Can you work these out from the model? Positions are in its coordinate system, mm. A direction names the side the tool comes from. Give positions to 0.01 mm unless a question says otherwise; leave off trailing zeros. Loops run counter-clockwise (first coordinate to the right, second up) from the corner with the lowest first, then second, coordinate; pieces in that order, holes last. Notation, with made-up numbers: (67.5, -13.5) - (77.5, -13.5) arc R24 ccw to (77.5, 1.5) - close; hole circle Ø5 at (73.25, 72). An arc over 180 degrees is marked (long way). Answer in a Markdown table with one row per item.
Autodesk Inventor part; units mm, degrees
ref_plane "YZ Plane" through (0, 0, 0) normal (1, 0, 0) x (0, 1, 0)
ref_plane "XZ Plane" through (0, 0, 0) normal (0, 1, 0) x (-1, 0, 0)
ref_plane "XY Plane" through (0, 0, 0) normal (0, 0, 1) x (1, 0, 0)
sketch "Sketch1" plane through (0, 0, 0) normal (1, 0, 0) x (0, 1, 0)
  line L0 (0, -278.2902) -> (0, 46.3817) construction
  line L1 (36.388, -206.3665) -> (0, 0) construction
  arc A0 (16.0424, -209.8254) -> (49.6755, -222.1573) centre (36.388, -206.3665) ccw
  line L2 (61.8586, -134.906) -> (45.7568, -169.4363) construction
  arc A1 (66.5803, -134.2844) -> (59.0717, -131.044) centre (61.8586, -134.906) ccw
  arc A2 (73.3134, -202.2667) -> (74.9688, -198.001) centre (70.247, -198.6226) ccw
  arc A3 (11.22, -165.5743) -> (9.3117, -170.2345) centre (14.0068, -169.4363) ccw
  line L3 (66.5803, -134.2844) -> (74.9688, -198.001)
  line L4 (73.3134, -202.2667) -> (49.6755, -222.1573)
  line L5 (16.0424, -209.8254) -> (9.3117, -170.2345)
  line L6 (70.247, -198.6226) -> (45.7568, -169.4363) construction
  line L7 (59.0717, -131.044) -> (11.22, -165.5743)
  line L8 (45.7568, -169.4363) -> (14.0068, -169.4363) construction
  dimension "d8" = 209.55
  dimension "d9" = 175.506
  dimension "d11" = 10
  dimension "d12" = 20.6375
  dimension "d13" = 38.1
  dimension "d14" = 25
  dimension "d19" = 4.7625
  dimension "d37" = 40
  dimension "d39" = 90
  dimension "d40" = 31.75
  dimension "d41" = 38.1
extrude "Plate1" add sketch "Sketch1" along normal blind 3.175
hole "Hole1" at (0, 61.8586, -134.906) at (0, 14.0068, -169.4363) at (0, 70.247, -198.6226) direction (1, 0, 0) diameter 4.9784 end through all
hole "Hole2" at (0, 36.388, -206.3665) at (0, 45.7568, -169.4363) direction (1, 0, 0) diameter 28.575 end through all
sketch "Sketch2" plane through (3.175, 0, 0) normal (1, 0, 0) x (0, 0, -1)
  circle A0 centre (169.4363, 45.7568) radius 14.2875
  circle A1 centre (206.3665, 36.388) radius 14.2875
  circle A2 centre (198.6226, 70.247) radius 2.4892
  circle A3 centre (169.4363, 14.0068) radius 2.4892
  circle A4 centre (134.906, 61.8586) radius 2.4892
  arc A5 (134.2844, 66.5803) -> (131.044, 59.0717) centre (134.906, 61.8586) ccw
  line L0 (165.5743, 11.22) -> (131.044, 59.0717)
  arc A6 (165.5743, 11.22) -> (170.2345, 9.3117) centre (169.4363, 14.0068) ccw
  line L1 (209.8254, 16.0424) -> (170.2345, 9.3117)
  arc A7 (209.8254, 16.0424) -> (222.1573, 49.6755) centre (206.3665, 36.388) ccw
  line L2 (202.2667, 73.3134) -> (222.1573, 49.6755)
  arc A8 (202.2667, 73.3134) -> (198.001, 74.9688) centre (198.6226, 70.247) ccw
  line L3 (134.2844, 66.5803) -> (198.001, 74.9688)
  line L4 (134.906, 61.8586) -> (198.6226, 70.247)
  line L5 (198.6226, 70.247) -> (218.5132, 46.6091)
  arc A9 (209.0271, 20.7375) -> (218.5132, 46.6091) centre (206.3665, 36.388) ccw
  line L6 (209.0271, 20.7375) -> (169.4363, 14.0068)
  line L7 (169.4363, 14.0068) -> (134.906, 61.8586)
  circle A10 centre (134.906, 61.8586) radius 4.7625
  circle A11 centre (198.6226, 70.247) radius 4.7625
  circle A12 centre (169.4363, 14.0068) radius 4.7625
  circle A13 centre (169.4363, 45.7568) radius 22.225
  circle A14 centre (206.3665, 36.388) radius 20.6375
  point P0 (0, 0)
  point P1 (196.0269, 18.5274)
  point P2 (186.3547, 31.3444)
  point P3 (161.5078, 24.9941)
  point P4 (166.6495, 17.8688)
  point P5 (174.1315, 14.805)
  point P6 (191.1791, 50.3612)
  point P7 (210.0229, 56.699)
  point P8 (201.689, 66.603)
  point P9 (193.9009, 69.6254)
  point P10 (175.3438, 67.1823)
  point P11 (147.233, 44.776)
  point P12 (158.1848, 64.9233)
  point P13 (139.6278, 62.4802)
  point P14 (137.6928, 57.9966)
  dimension "d42" = 4.7625
  dimension "d44" = 41.275
  dimension "d45" = 44.45
extrude "Cut1" cut sketch "Sketch2" against normal blind 3.175 contours A11 L5 A14 A13 L4 | A13 L7 A10 L4 | A14 L6 A12 L7 A13
fillet "Corner Round1" radius 1.5875 14 edges at (1.5875, 44.776, -147.233) (1.5875, 64.9233, -158.1848) (1.5875, 57.9966, -137.6928) (1.5875, 56.699, -210.0229) (1.5875, 31.3444, -186.3547) (1.5875, 14.805, -174.1315) (1.5875, 18.5274, -196.0269) (1.5875, 50.3612, -191.1791) (1.5875, 62.4802, -139.6278) (1.5875, 69.6254, -193.9009) (1.5875, 66.603, -201.689) (1.5875, 67.1823, -175.3438) (1.5875, 17.8688, -166.6495) (1.5875, 24.9941, -161.5078)
equation "\"d25\" = Thickness"
equation "\"d46\" = Thickness"
equation "\"d7\" = Thickness"
equation "\"BendRadius\" = Thickness"
equation "\"BendReliefWidth\" = Thickness"
equation "\"BendReliefDepth\" = 0.5 * Thickness"
equation "\"CornerReliefSize\" = 4 * Thickness"
equation "\"MinimumRemnant\" = 2 * Thickness"
equation "\"TransitionRadius\" = BendRadius"
equation "\"JacobiRadiusSize\" = BendRadius"
equation "\"GapSize\" = Thickness"
properties part number "PLATE,BEARING,MOUNT" material "Aluminum 3003-H16"
Q1. If we mould it in two halves opening along Y, with no side actions, what happens to faces 1 (the face through (3.175, 42, -189)), 2 (the face through (1.565, 18.395, -166.691)), 3 (the face through (1.57, 74.7, -200.31))? For each: released by +Y, released by -Y, zero draft, split by the parting line, or undercut.
Checked values:
| item | result |
|---|---|
| face 1 | zero draft |
| face 2 | undercut |
| face 3 | released by +Y |
Q2. Imagine slicing it at A-A, the plane z = -176.5. Write out the boundary of the cut face in (x, y) (3 decimals).
Checked values:
| item | result |
|---|---|
| outline | (0, 10.377) - (3.175, 10.377) - (3.175, 15.208) - (0, 15.208) - close; (0, 24.684) - (3.175, 24.684) - (3.175, 33.338) - (0, 33.338) - close; (0, 58.176) - (3.175, 58.176) - (3.175, 72.138) - (0, 72.138) - close |
Q3. For pin 1 (1 mm diameter, centred on x = 1.5, z = -190.5, fed in from -Y); pin 2 (5 mm diameter, centred on y = 28, z = -196, fed in from +X) (3 decimals); pin 3 (1 mm diameter, centred on x = 0.5, z = -190, fed in from +Y); pin 4 (17 mm diameter, centred on y = 45.76, z = -169.44, fed in from +X), each with a flat end and sliding along its axis, tell me the tip position at first contact or that it passes through.
Checked values:
| item | result |
|---|---|
| pin 1 | stops at y = 12.67 |
| pin 2 | stops at x = 3.175 |
| pin 3 | stops at y = 73.98 |
| pin 4 | passes through |
Q4. If I drill on line 1 (Y direction, x = 0.3, z = -169); line 2 (Z direction, x = 2.7, y = 52); line 3 (Y direction, x = 0.2, z = -200), over which ranges is the centre line in solid material (lowest first)? Write a range as [from, to].
Checked values:
| item | result |
|---|---|
| line 1 | y = [9.26, 11.56], [16.46, 18.75], [23.54, 31.48], [60.04, 71.15] |
| line 2 | z = [-220.2, -192.84], [-191.17, -182.29], [-156.59, -148.11], [-142.02, -136.15] |
| line 3 | y = [14.37, 23.6], [49.18, 56.02], [65.69, 68.17], [72.32, 74.81] |
Q5. Imagine slicing it at B-B, the plane y = 38. Write out the boundary of the cut face in (x, z) (3 decimals).
Checked values:
| item | result |
|---|---|
| outline | (0, -226.941) - (3.175, -226.941) - (3.175, -220.563) - (0, -220.563) - close; (0, -192.17) - (3.175, -192.17) - (3.175, -181.435) - (0, -181.435) - close; (0, -157.438) - (3.175, -157.438) - (3.175, -146.25) - (0, -146.25) - close |
Q6. On a 3-axis mill with a long thin cutter (end or side, diameter ignored), from which of +Z, -Z, +X, -X, +Y, -Y can I reach the whole of each face in a straight line? I mean faces 4 (the face through (1.61, 52.58, -141.6)), 5 (the face through (0, 42, -189)). Say none if no direction works.
Checked values:
| item | result |
|---|---|
| face 4 | +X, -X |
| face 5 | +Z, -Z, -X, +Y, -Y |
Q7. Imagine slicing it at C-C, the plane x = 2.6. Count the separate pieces of the cut face and the enclosed holes in it, and give its area (3 significant figures).
Checked values:
| item | result |
|---|---|
| separate pieces | 1 |
| enclosed holes | 8 |
| area | 2,380 mm² |
